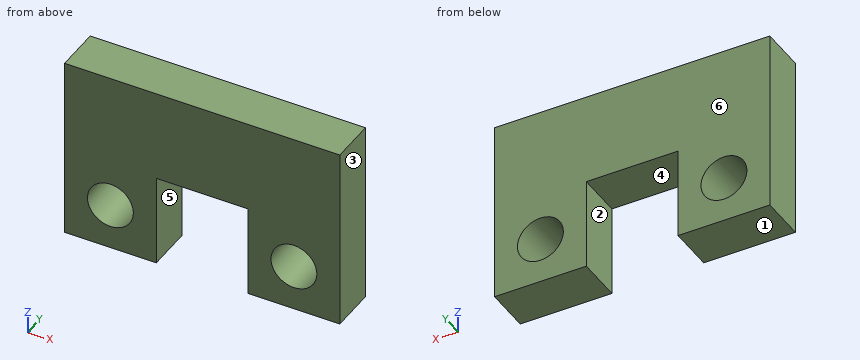
```python
from build123d import *

# Parameters (mm, degrees)
BOSS_EXTRUDE1_DEPTH = 20
SKETCH4_R           = 10
CUT_EXTRUDE1_DEPTH  = 20


with BuildPart() as part:
    # Sketch2 → Boss-Extrude1 (new body)
    with BuildSketch(Plane(origin=(0, 0, 0), x_dir=(1, 0, 0), z_dir=(0, 1, 0))):
        Polygon((0, 0), (120, 0), (120, 80), (80, 80), (80, 40), (40, 40), (40, 80), (0, 80), align=None)
    extrude(amount=BOSS_EXTRUDE1_DEPTH)

    # Sketch4 → Cut-Extrude1 (cut)
    with BuildSketch(Plane.XZ):
        with Locations((20, -60)):
            Circle(SKETCH4_R)
        with Locations((100, -60)):
            Circle(SKETCH4_R)
    extrude(amount=-CUT_EXTRUDE1_DEPTH, mode=Mode.SUBTRACT)


solid = part.part
```
Design review of the part built by this model. Coordinates are the model's own, in mm. Face numbers are marked on the shaded views. A direction names the side the tool comes from. Coordinates: 2 decimals unless noted, no trailing zeros. Order: outer loops, then holes, each group sorted by start corner. A loop starts at its lowest first (then second) coordinate and runs counter-clockwise, first axis right, second up. Notation, with made-up numbers: (69.5, 79) - (125.5, 79) arc R27 ccw to (125.5, 106) - close; hole circle Ø8 at (-23, -17). An arc over 180 degrees is marked (long way). One line per question, with ' | ' between items.
Q1. To check wall thickness, follow line 1 along Z through (x, y) = (20, 13.75); line 2 along X through (y, z) = (19, -45.5); line 3 along Z through (x, y) = (108, 6). State the ranges of each line that lie inside material, in increasing order.
Answer key:
line 1: z = -80 to -70, -50 to 0 | line 2: x = 0 to 40, 80 to 120 | line 3: z = -80 to -66, -54 to 0
Q2. For the marked faces 5 and 6, list the 3-axis set-ups (+Z, -Z, +X, -X, +Y, -Y) from which the entire face can be reached by the end or side of a thin tool; tool diameter is ignored.
Answer key:
face 5: -Z, +Y, -Y | face 6: +Z, -Z, +X, -X, +Y
Q3. Clearance check with a flat-ended pin moving along its axis: pin 1 Ø10 at (x, y) = (51, 7.5) entering from -Z. State where the tip first meets the part, or that it passes through.
Answer key:
pin 1: stops at z = -40
Q4. Consider section B-B, the plane x = 20. Give the boundary of the cut face in (y, z).
Answer key:
outline: (0, -80) - (20, -80) - (20, -70) - (0, -70) - close; (0, -50) - (20, -50) - (20, 0) - (0, 0) - close
Q5. Consider section A-A, the plane z = -60. Give the boundary of the cut face in (x, y).
Answer key:
outline: (0, 0) - (10, 0) - (10, 20) - (0, 20) - close; (30, 0) - (40, 0) - (40, 20) - (30, 20) - close; (80, 0) - (90, 0) - (90, 20) - (80, 20) - close; (110, 0) - (120, 0) - (120, 20) - (110, 20) - close
Q6. Consider section C-C, the plane y = 9. Give the boundary of the cut face in (x, z), then the cut area to 3 significant figures.
Answer key:
outline: (0, -80) - (40, -80) - (40, -40) - (80, -40) - (80, -80) - (120, -80) - (120, 0) - (0, 0) - close; hole circle Ø20 at (20, -60); hole circle Ø20 at (100, -60) | area: 7,370 mm2
Q7. The part is to be moulded in two halves that separate along X. For the marked faces 1, 2, 3 and 4, say which applies: +X half, -X half, draft (parallel to the pull), parting line (faces both ways), or undercut.
Answer key:
face 1: draft | face 2: undercut | face 3: +X half | face 4: undercut
Q8. Consider section D-D, the plane z = -75. Give the boundary of the cut face in (x, y), then the cut area to 3 significant figures.
Answer key:
outline: (0, 0) - (40, 0) - (40, 20) - (0, 20) - close; (80, 0) - (120, 0) - (120, 20) - (80, 20) - close | area: 1,600 mm2
